```python
from build123d import *

# Parameters (mm, degrees)
SKETCH1_W             = 4
SKETCH1_H             = 7
BOSS_EXTRUDE1_DEPTH   = 24
BOSS_EXTRUDE1_2_DEPTH = 24
BOSS_EXTRUDE2_START   = 20
SKETCH1_3_W           = 20
SKETCH1_3_H           = 7
BOSS_EXTRUDE2_DEPTH   = 4
SKETCH2_W             = 8
SKETCH2_H             = 2.193366053
BOSS_EXTRUDE3_DEPTH   = 70
SKETCH3_W             = 8
SKETCH3_H             = 8.193366053
BOSS_EXTRUDE4_DEPTH   = 4
CUT_EXTRUDE1_REACH    = 100.423
SKETCH4_R             = 1.65
CHAMFER1_SIZE         = 13
SKETCH5_W             = 8
SKETCH5_H             = 74
BOSS_EXTRUDE5_DEPTH   = 1


with BuildPart() as part:
    # Sketch1 → Boss-Extrude1 (new body)
    with BuildSketch(Plane.XY):
        with Locations((-2, 3.5)):
            Rectangle(SKETCH1_W, SKETCH1_H)
    extrude(amount=BOSS_EXTRUDE1_DEPTH)



with BuildPart() as body_2:
    # Sketch1 → Boss-Extrude1 2 (new body)
    with BuildSketch(Plane.XY):
        with Locations((22, 3.5)):
            Rectangle(SKETCH1_W, SKETCH1_H)
    extrude(amount=BOSS_EXTRUDE1_2_DEPTH)


with BuildPart() as part_1:
    add(part.part)

    add(body_2.part)  # Boss-Extrude2 merges body 2
    # Sketch1<3> → Boss-Extrude2 (add)
    with BuildSketch(Plane.XY.offset(BOSS_EXTRUDE2_START)):
        with Locations((10, 3.5)):
            Rectangle(SKETCH1_3_W, SKETCH1_3_H)
    extrude(amount=BOSS_EXTRUDE2_DEPTH)



with BuildPart() as body_2_2:
    # Sketch2 → Boss-Extrude3 (new body)
    with BuildSketch(Plane.XY.offset(24)):
        with Locations((10, -7.096683027)):
            Rectangle(SKETCH2_W, SKETCH2_H)
    extrude(amount=BOSS_EXTRUDE3_DEPTH)


with BuildPart() as part_2:
    add(part_1.part)

    add(body_2_2.part)  # Boss-Extrude4 merges body 2 2
    # Sketch3 → Boss-Extrude4 (add)
    with BuildSketch(Plane(origin=(0, 0, 24), x_dir=(-1, 0, 0), z_dir=(0, 0, -1))):
        with Locations((-10, -4.096683027)):
            Rectangle(SKETCH3_W, SKETCH3_H)
    extrude(amount=BOSS_EXTRUDE4_DEPTH)

    # Cut-Extrude1: up to this face of the body (flat: up to its plane)
    cut_extrude1_end = Plane(part_2.part.faces().sort_by_distance((-4, 3.5, 12))[0])
    # Sketch4 → Cut-Extrude1 (cut, up to the picked face)
    with BuildSketch(Plane(origin=(24, 0, 0), x_dir=(0, 0, -1), z_dir=(1, 0, 0)), mode=Mode.PRIVATE) as cut_extrude1_sk1:
        with Locations((-10, 3.5)):
            Circle(SKETCH4_R)
    cut_extrude1_tool1 = split(extrude(cut_extrude1_sk1.sketch, amount=-CUT_EXTRUDE1_REACH, mode=Mode.PRIVATE), bisect_by=cut_extrude1_end, keep=Keep.BOTH, mode=Mode.PRIVATE)
    add(cut_extrude1_tool1.solids().sort_by(Axis((24, 3.5, 10), (-1, 0, 0)))[0], mode=Mode.SUBTRACT)

    # Chamfer1
    chamfer1_edges = [part_2.edges().sort_by_distance(p)[0] for p in [
        (10, -6, 24),
    ]]
    chamfer(chamfer1_edges, length=CHAMFER1_SIZE - 0.0001)  # a hair under: the kernel refuses the full size

    # Sketch5 → Boss-Extrude5 (add)
    with BuildSketch(Plane.XZ.offset(8.193366053)):
        with Locations((10, 57)):
            Rectangle(SKETCH5_W, SKETCH5_H)
    extrude(amount=BOSS_EXTRUDE5_DEPTH)


solid = part_2.part
```
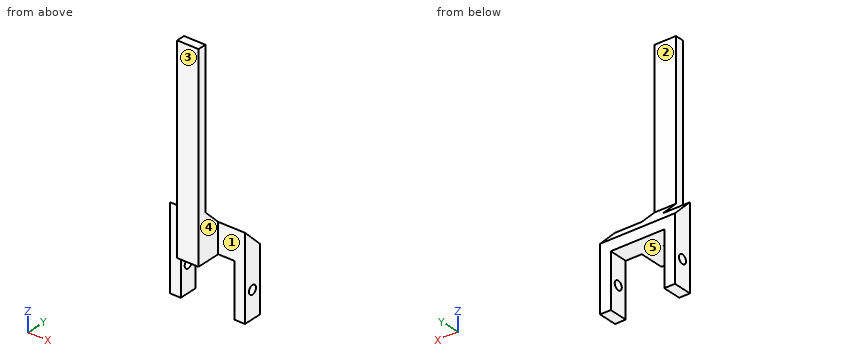
CAD build for the part. Positions are in the model's coordinates, mm. Face numbers are marked on the shaded views. A direction names the side the tool comes from. Give positions to 0.01 mm unless a question says otherwise; leave off trailing zeros. Loops run counter-clockwise (first coordinate to the right, second up) from the corner with the lowest first, then second, coordinate; pieces in that order, holes last. Notation, with made-up numbers: (0.5, -10) - (28.5, -10) arc R8 cw to (28.5, -4) - close; hole circle Ø6 at (-6, 88). An arc over 180 degrees is marked (long way). Put each result on its own line as item: value.
Q1. Probe line 1 along Y through (x, z) = (22.3, 10); line 2 along Z through (x, y) = (3, 6.25); line 3 along Y through (x, z) = (5.5, 28). List the from-to ranges inside material, lowest first.
Filled in:
line 1: y = 0 to 1.85, 5.15 to 7
line 2: z = 20 to 24.75
line 3: y = 0 to 3
Q2. Slice it at D-D (z = 67.5). Give the cut face in (x, y).
Filled in:
outline: (6, -9.19) - (14, -9.19) - (14, -6) - (6, -6) - close
Q3. Slice it at C-C (y = 3.5). Give the cut face in (x, z).
Filled in:
outline: (-4, 0) - (0, 0) - (0, 8.35) - (-4, 8.35) - close; (-4, 11.65) - (0, 11.65) - (0, 20) - (20, 20) - (20, 11.65) - (24, 11.65) - (24, 27.5) - (-4, 27.5) - close; (20, 0) - (24, 0) - (24, 8.35) - (20, 8.35) - close
Q4. Flat gauge pins, fed straight in: pin 1 (3 mm diameter, centred on x = 20, z = 27, fed in from +Y); pin 2 (8 mm diameter, centred on x = 7.5, y = 5.5, fed in from +Z); pin 3 (3 mm diameter, centred on x = 1, y = 2, fed in from -Z); pin 4 (6.5 mm diameter, centred on x = 9.5, z = 77, fed in from +Y). Where does each tip first touch, or does it go through?
Filled in:
pin 1: stops at y = 5.5
pin 2: stops at z = 29.5
pin 3: stops at z = 0
pin 4: stops at y = -6
Q5. Tool access for the marked faces 1 and 2: list every direction of +Z, -Z, +X, -X, +Y, -Y with a clear straight run to the whole face (end or side of a thin tool).
Filled in:
face 1: +Z, -Z, +X, -Y
face 2: +Z, +X, -X, +Y
Q6. Slice it at A-A (z = 18). Give the cut face in (x, y), plus the area to 3 significant figures.
Filled in:
outline: (-4, 0) - (0, 0) - (0, 7) - (-4, 7) - close; (20, 0) - (24, 0) - (24, 7) - (20, 7) - close
area: 56.0 mm²
Q7. Mould opens along X. For the marked faces 3, 4 and 5 say: pulls with the +X half, pulls with the -X half, needs draft (parallel to the pull), parting line crosses it, or undercut.
Filled in:
face 3: needs draft
face 4: pulls with the +X half
face 5: undercut
